Here's how the part is built. I have some questions about the finished solid (model axes, mm). Face numbers are marked on the shaded views. A direction names the side the tool comes from. Coordinates: 2 decimals unless noted, no trailing zeros. Write each loop counter-clockwise with the first axis right and the second up, starting at its lowest first coordinate (ties: lowest second). Pieces come first, ordered by that corner, then holes. Notation, with made-up numbers: (-0.75, 82.25) -> (41.25, 82.25) arc R26 ccw to (41.25, 105.25) -> close; hole circle Ø6 at (41, 74). An arc over 180 degrees is marked (long way). Put each result on its own line as item: value.
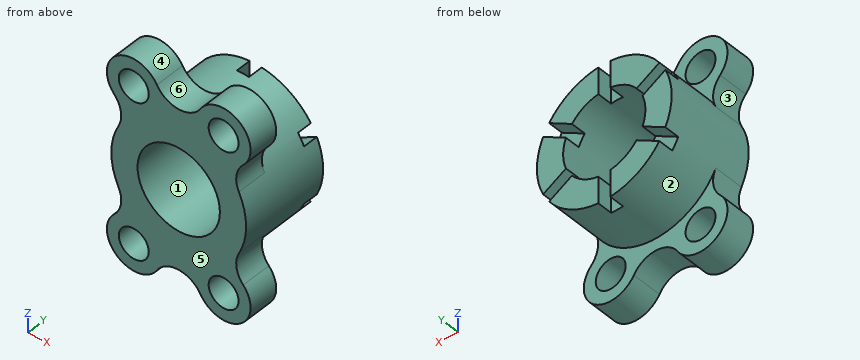
Autodesk Fusion 360 part; units mm, degrees
sketch "Sketch1" plane through (0, 0, 0) normal (0, 1, 0) x (1, 0, 0)
  circle A0 centre (0, 0) radius 27.5
  circle A1 centre (0, 0) radius 45
  line L0 (0, 0) -> (110, 0) construction
  line L1 (0, 0) -> (0, 75) construction
  line L2 (0, 0) -> (-52.945, 91.7035) construction
  line L3 (0, 0) -> (105.89, 0) construction
  circle A2 centre (-30, 51.9615) radius 10
  circle A3 centre (30, 51.9615) radius 10
  arc A4 (-14.5714, 61.2329) -> (14.5714, 61.2329) centre (0, 69.9893) ccw
  arc A5 (-40.1988, 20.2252) -> (-43.0551, 39.5694) centre (-55.385, 27.8658) ccw
  arc A6 (43.0551, 39.5694) -> (40.1988, 20.2252) centre (55.385, 27.8658) ccw
  arc A7 (-14.5714, 61.2329) -> (-43.0551, 39.5694) centre (-30, 51.9615) ccw
  arc A8 (43.0551, 39.5694) -> (14.5714, 61.2329) centre (30, 51.9615) ccw
  arc A9 (-43.0551, -39.5694) -> (-40.1988, -20.2252) centre (-55.385, -27.8658) ccw
  arc A10 (-43.0551, -39.5694) -> (-14.5714, -61.2329) centre (-30, -51.9615) ccw
  arc A11 (14.5714, -61.2329) -> (-14.5714, -61.2329) centre (0, -69.9893) ccw
  arc A12 (14.5714, -61.2329) -> (43.0551, -39.5694) centre (30, -51.9615) ccw
  arc A13 (40.1988, -20.2252) -> (43.0551, -39.5694) centre (55.385, -27.8658) ccw
  circle A14 centre (30, -51.9615) radius 10
  circle A15 centre (-30, -51.9615) radius 10
  dimension "d1" = 55
  dimension "d2" = 90
  dimension "d3" = 120
  dimension "d4" = 20
  dimension "d5" = 36
  dimension "d6" = 60
  dimension "d7" = 17
  dimension "d8" = 17
  dimension "d9" = 17
extrude "Extrude1" add sketch "Sketch1" along normal blind 20 contours A1 A4 A5 A6 A7 A8 | A1 A9 A10 A11 A12 A13 makes body 1 at (39.1578, 13.3333, 22.1736) makes body 2 at (39.1578, 6.6667, -22.1736)
extrude "Extrude2" add sketch "Sketch1" along normal blind 60 contours A1 bodies 1 2
sketch "Sketch2" plane through (0, 60, 0) normal (0, 1, 0) x (-1, 0, 0)
  circle A0 centre (0, 0) radius 27.5
  circle A1 centre (0, 0) radius 45
  line L0 (-4, -22.5) -> (4, -22.5)
  line L1 (4, -22.5) -> (4, -47.5)
  line L2 (4, -47.5) -> (-4, -47.5)
  line L3 (-4, -47.5) -> (-4, -22.5)
  line L4 (-4, -22.5) -> (4, -47.5) construction
  line L5 (4, -22.5) -> (-4, -47.5) construction
  point P0 (0, -35)
  dimension "d14" = 8
  dimension "d15" = 25
extrude "Extrude3" cut sketch "Sketch2" against normal blind 10 contours A0 A1 L1 L3 picked at (-3.1125, -33.1656) bodies 1
pattern_circular "C-Pattern1" count 6 over 360 about axis through (0, 60, 0) along (0, -1, 0) of "Extrude3"
Item 1: Imagine slicing it at A-A on z = 0. Write out the boundary of the cut face in (x, y), then the cut area to 3 significant figures.
Output:
outline: (-45, 0) -> (-27.5, 0) -> (-27.5, 60) -> (-45, 60) -> close; (27.5, 0) -> (45, 0) -> (45, 60) -> (27.5, 60) -> close
area: 2,100 mm²
Item 2: If we mould it in two halves opening along X, with no side actions, what happens to the marked faces 3, 4, 5 and 6? For each: released by +X, released by -X, zero draft, split by the parting line, or undercut.
Output:
face 3: released by -X
face 4: undercut
face 5: zero draft
face 6: undercut
Item 3: For P1, Ø2, axis at x = 9.5, y = 11.5, coming from the -Z side; P2, Ø1.5, axis at y = 14.5, z = 44.5, coming from the +X side; P3, Ø16, axis at x = 30, z = -51.96, coming from the -Y side; P4, Ø5, axis at y = 56.5, z = 34, coming from the -X side, each with a flat end and sliding along its axis, tell me the tip position at first contact or that it passes through.
Output:
P1: stops at z = -56.62
P2: stops at x = 46.7
P3: passes through
P4: stops at x = -32.14
Item 4: Please list where these lines run through material, in increasing order: line 1 along X through (y, z) = (10.5, 51.5); line 2 along Z through (x, y) = (30, 13); line 3 along X through (y, z) = (47, 0). Write a range as from..to.
Output:
line 1: x = -47.99..-39.99, -20.01..20.01, 39.99..47.99
line 2: z = -69.96..-61.96, -41.96..41.96, 61.96..69.96
line 3: x = -45..-27.5, 27.5..45
Item 5: Imagine slicing it at D-D on y = 34. Write out the boundary of the cut face in (x, z), then the cut area to 3 significant figures.
Output:
outline: circle Ø90 at (0, 0); hole circle Ø55 at (0, 0)
area: 3,990 mm²
Item 6: Imagine slicing it at C-C on x = -30. Write out the boundary of the cut face in (y, z), then the cut area to 3 significant figures.
Output:
outline: (0, -69.96) -> (20, -69.96) -> (20, -61.96) -> (0, -61.96) -> close; (0, -41.96) -> (20, -41.96) -> (20, -33.54) -> (60, -33.54) -> (60, -21.94) -> (50, -21.94) -> (50, -12.7) -> (60, -12.7) -> (60, 12.7) -> (50, 12.7) -> (50, 21.94) -> (60, 21.94) -> (60, 33.54) -> (20, 33.54) -> (20, 41.96) -> (0, 41.96) -> close; (0, 61.96) -> (20, 61.96) -> (20, 69.96) -> (0, 69.96) -> close
area: 4,500 mm²
Item 7: Imagine slicing it at B-B on x = 0. Write out the boundary of the cut face in (y, z), then the cut area to 3 significant figures.
Output:
outline: (0, -52.99) -> (20, -52.99) -> (20, -45) -> (50, -45) -> (50, -27.5) -> (0, -27.5) -> close; (0, 27.5) -> (50, 27.5) -> (50, 45) -> (20, 45) -> (20, 52.99) -> (0, 52.99) -> close
area: 2,070 mm²
Item 8: Which directions (+Z, -Z, +X, -X, +Y, -Y) give clear straight access to the entire face, cutting with the end or side of a thin tool? Please do the marked faces 1 and 2.
Output:
face 1: +Y, -Y
face 2: +Y
